For this review, take the finished solid that the model builds, in its own axes (mm). Coordinates: 2 decimals unless noted, no trailing zeros. Write each loop counter-clockwise with the first axis right and the second up, starting at its lowest first coordinate (ties: lowest second). Pieces come first, ordered by that corner, then holes. Notation, with made-up numbers: M -16,-0.5 L 14,-0.5 A15 ccw 14,3.5 Z; hole C 23,66 d9. An arc over 180 degrees is marked long. One line per question, with ' | ' between items.
from build123d import *

# Parameters (mm, degrees)
SKETCH1_R           = 87.5
BOSS_EXTRUDE1_DEPTH = 3.18
SKETCH2_W           = 7
SKETCH2_H           = 35
CUT_EXTRUDE1_DEPTH  = 3.18
SKETCH7_R           = 2.95
CUT_EXTRUDE5_DEPTH  = 10
SKETCH8_R           = 1.47
CUT_EXTRUDE6_DEPTH  = 124.78454023
SKETCH3_W           = 3.18
SKETCH3_H           = 8
CUT_EXTRUDE13_DEPTH = 124.78454023


with BuildPart() as part:
    # Sketch1 → Boss-Extrude1 (new body)
    with BuildSketch(Plane(origin=(0, 0, 0), x_dir=(1, 0, 0), z_dir=(0, 1, 0))):
        with Locations(Location((0, 0, 0), (0, 0, 90))):
            Circle(SKETCH1_R)
    extrude(amount=BOSS_EXTRUDE1_DEPTH)

    # Sketch2 → Cut-Extrude1 (cut)
    with BuildSketch(Plane(origin=(0, 3.18, 0), x_dir=(1, 0, 0), z_dir=(0, 1, 0))):
        with Locations((-40, 0)):
            Rectangle(SKETCH2_W, SKETCH2_H)
        with Locations((40, 0)):
            Rectangle(SKETCH2_W, SKETCH2_H)
    extrude(amount=-CUT_EXTRUDE1_DEPTH, mode=Mode.SUBTRACT)

    # Sketch7 → Cut-Extrude5 (cut)
    with BuildSketch(Plane.XZ):
        with Locations(Location((0, 0, 0), (0, 0, 270))):
            Circle(SKETCH7_R)
    extrude(amount=-CUT_EXTRUDE5_DEPTH, mode=Mode.SUBTRACT)

    # Sketch8 → Cut-Extrude6 (cut, through all)
    with BuildSketch(Plane(origin=(0, 3.18, 0), x_dir=(1, 0, 0), z_dir=(0, 1, 0))):
        with Locations(Location((0, 13.975, 0), (0, 0, 270))):
            Circle(SKETCH8_R)
        with Locations(Location((0, -13.975, 0), (0, 0, 270))):
            Circle(SKETCH8_R)
    extrude(amount=-CUT_EXTRUDE6_DEPTH, mode=Mode.SUBTRACT)

    # Sketch3 → Cut-Extrude13 (cut, through all)
    with BuildSketch(Plane.XZ):
        with Locations((56.29, -13.84)):
            Rectangle(SKETCH3_W, SKETCH3_H)
        with Locations((56.29, 35.66)):
            Rectangle(SKETCH3_W, SKETCH3_H)
        with Locations((-56.29, 13.84)):
            Rectangle(SKETCH3_W, SKETCH3_H)
        with Locations((-56.29, -35.66)):
            Rectangle(SKETCH3_W, SKETCH3_H)
    extrude(amount=-CUT_EXTRUDE13_DEPTH, mode=Mode.SUBTRACT)


solid = part.part
1. Draft analysis for pull direction X (two halves, no side actions). For faces 1 (the flat face through (-1, 3.18, -18)), 2 (the cylindrical face through (-2.88, 1.57, 0.64)), 3 (the cylindrical face through (-86.755, 1.568, 11.391)), state which applies: pulls with the +X half, pulls with the -X half, needs draft (parallel to the pull), parting line crosses it, or undercut.
Computed values:
face 1: needs draft | face 2: undercut | face 3: parting line crosses it
2. Take a section at B-B on y = 2.35. Give the number of separate pieces and of enclosed holes in the cut face, plus the area to 3 significant figures.
Computed values:
separate pieces: 1 | enclosed holes: 9 | area: 23,400 mm2
3. For line 1 along X through (y, z) = (0.25, 0); line 2 along X through (y, z) = (1.4, -15); line 3 along X through (y, z) = (1.6, -1), list the stretches that pass through material, from the lowest coordinate up.
Computed values:
line 1: x = -87.5 to -43.5, -36.5 to -2.95, 2.95 to 36.5, 43.5 to 87.5 | line 2: x = -86.2 to -43.5, -36.5 to -1.05, 1.05 to 36.5, 43.5 to 54.7, 57.88 to 86.2 | line 3: x = -87.49 to -43.5, -36.5 to -2.78, 2.78 to 36.5, 43.5 to 87.49
4. Take a section at A-A on z = 0. State the section outline as (x, y) points, plus the area to 3 significant figures.
Computed values:
outline: M -87.5,0 L -43.5,0 L -43.5,3.18 L -87.5,3.18 Z; M -36.5,0 L -2.95,0 L -2.95,3.18 L -36.5,3.18 Z; M 2.95,0 L 36.5,0 L 36.5,3.18 L 2.95,3.18 Z; M 43.5,0 L 87.5,0 L 87.5,3.18 L 43.5,3.18 Z | area: 493 mm2
5. Clearance check with flat-ended pins moving along their axes: P1, Ø1.6, axis at y = 2, z = 36.5, coming from the +X side; P2, Ø1, axis at x = -39.5, y = 1, coming from the +Z side; P3, Ø1.6, axis at x = -56, y = 1, coming from the -Z side. State where each tip first meets the part, or that it passes through.
Computed values:
P1: stops at x = 79.89 | P2: stops at z = 78.33 | P3: stops at z = -67.89
6. Take a section at C-C on z = 36.5. State the section outline as (x, y) points, plus the area to 3 significant figures.
Computed values:
outline: M -79.52,0 L 54.7,0 L 54.7,3.18 L -79.52,3.18 Z; M 57.88,0 L 79.52,0 L 79.52,3.18 L 57.88,3.18 Z | area: 496 mm2
7. Take a section at D-D on x = 39.5. State the section outline as (y, z) points, plus the area to 3 significant figures.
Computed values:
outline: M 0,-78.08 L 3.18,-78.08 L 3.18,-17.5 L 0,-17.5 Z; M 0,17.5 L 3.18,17.5 L 3.18,78.08 L 0,78.08 Z | area: 385 mm2
